Read the model definition and answer for the solid it produces. Units are mm, in the model's axes. Face numbers are marked on the shaded views. A direction names the side the tool comes from. Coordinates: 2 decimals unless noted, no trailing zeros. Write each loop counter-clockwise with the first axis right and the second up, starting at its lowest first coordinate (ties: lowest second). Pieces come first, ordered by that corner, then holes.
(1) Which of the six approach directions +Z, -Z, +X, -X, +Y, -Y give full straight-line access (tool end or side, diameter ignored) to the marked faces 1, 2 and 3?
(2) Given pin 1 (2 mm diameter, centred on x = 34, z = 3.5, fed in from +Y); pin 2 (2 mm diameter, centred on y = 5.5, z = 0, fed in from +X); pin 3 (12 mm diameter, centred on x = 62.5, y = -2, fed in from +Z) (3 decimals), each flat-ended and moving along its own axis, determine where each tip first touches the part or whether it passes through.
(3) The part is cut by section C-C, the plane x = 58. Determine the outline of the cut face in (y, z) (3 decimals), and give its area (3 significant figures).
(4) Straight lines are drawn through the part: line 1 along X through (y, z) = (-4.25, -0.25); line 2 along Y through (x, z) = (13, 0) (3 decimals); line 3 along Y through (x, z) = (126, 2.5). For each, find the intervals that lie inside material, in ascending order.
(5) The part is cut by section D-D, the plane z = 9.25. Determine the outline of the cut face in (x, y), and give its area (3 significant figures).
```python
from build123d import *

# Parameters (mm, degrees)
SKETCH3_W = 76.9874
SKETCH3_H = 3.175
SKETCH5_W = 0.254
SKETCH5_H = 0.508
SKETCH6_W = 0.254
SKETCH6_H = 0.508


with BuildPart() as part:
    # Sketch1 → Revolve1 (revolve)
    with BuildSketch(Plane.XY):
        Polygon((0, 0), (0, 3.175), (76.9874, 3.175), (76.9874, 11.19505), (98.5266, 11.19505), (98.5266, 0), align=None)
    revolve(axis=Axis((98.5266, 0, 0), (-1, 0, 0)))

    # Sketch2 → Revolve2 (revolve)
    with BuildSketch(Plane.XY):
        Polygon((-12.7, 0), (-12.7, 2.63398), (-12.15898, 3.175), (0, 3.175), (0, 0), align=None)
    revolve(axis=Axis((0, 0, 0), (-1, 0, 0)))

    # Sketch3 → Revolve3 (revolve)
    with BuildSketch(Plane.XY):
        with Locations((137.0203, 1.5875)):
            Rectangle(SKETCH3_W, SKETCH3_H)
    revolve(axis=Axis((175.514, 0, 0), (-1, 0, 0)))

    # Sketch4 → Revolve4 (revolve)
    with BuildSketch(Plane.XY):
        Polygon((175.514, 0), (175.514, 3.175), (187.67298, 3.175), (188.214, 2.63398), (188.214, 0), align=None)
    revolve(axis=Axis((188.214, 0, 0), (-1, 0, 0)))

    # Sketch5 → Cut-Revolve1 (revolve, cut)
    with BuildSketch(Plane.XY):
        with Locations((-0.127, 3.175)):
            Rectangle(SKETCH5_W, SKETCH5_H)
    revolve(axis=Axis((0, 0, 0), (-1, 0, 0)), mode=Mode.SUBTRACT)

    # Sketch6 → Cut-Revolve2 (revolve, cut)
    with BuildSketch(Plane.XY):
        with Locations((175.641, 3.175)):
            Rectangle(SKETCH6_W, SKETCH6_H)
    revolve(axis=Axis((175.768, 0, 0), (-1, 0, 0)), mode=Mode.SUBTRACT)


solid = part.part
```
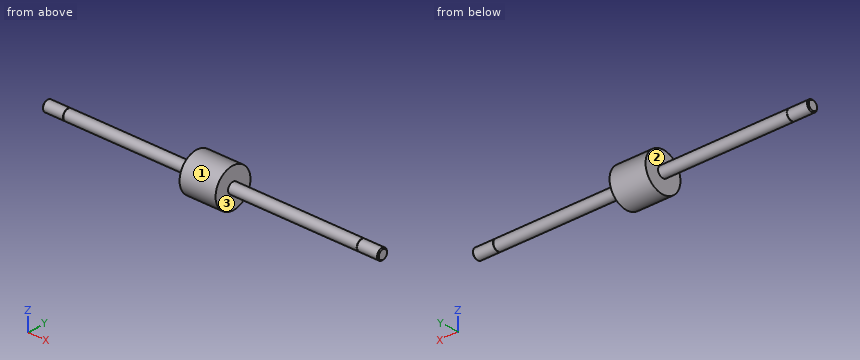
Computed:
1. face 1: +X, -X
1. face 2: -X
1. face 3: +X
2. pin 1: stops at y = 1.96
2. pin 2: stops at x = 98.53
2. pin 3: stops at z = 3.175
3. outline: circle Ø6.35 at (0, 0)
3. area: 31.7 mm2
4. line 1: x = 76.99 to 98.53
4. line 2: y = -3.175 to 3.175
4. line 3: y = -1.96 to 1.96
5. outline: (76.99, -6.31) - (98.53, -6.31) - (98.53, 6.31) - (76.99, 6.31) - close
5. area: 272 mm2
